The listing builds one solid part. Answer for the finished solid, in the listing's coordinates (mm). Face numbers are marked on the shaded views. A direction names the side the tool comes from. Give positions to 0.01 mm unless a question says otherwise; leave off trailing zeros. Write each loop counter-clockwise with the first axis right and the second up, starting at its lowest first coordinate (ties: lowest second). Pieces come first, ordered by that corner, then holes. Notation, with made-up numbers: (43.25, 17.25) - (91.25, 17.25) arc R26 cw to (91.25, 42.25) - close; hole circle Ø9 at (8, 49.25). An arc over 180 degrees is marked (long way). One line per question, with ' | ' between items. Start each with the question number.
1. Given P1, Ø5, axis at x = -9.5, y = -34, coming from the -Z side; P2, Ø9.5, axis at x = -35, y = -20.5, coming from the +Z side; P3, Ø2, axis at x = -29.5, z = 50.5, coming from the +Y side; P4, Ø8.5, axis at x = -37.99, y = 13.53, coming from the +Z side, each flat-ended and moving along its own axis, determine where each tip first touches the part or whether it passes through.
2. The mould has two halves that part along X. Classify the marked faces 3, 4 and 5: +X half, -X half, draft (parallel to the pull), parting line (faces both ways), or undercut.
3. A cutting plane is placed at A-A (y = 26). Determine the outline of the cut face in (x, z).
4. Find the intervals of material crossed by L1, parallel to Z at x = -31, y = -11.5; L2, parallel to Y at x = -6, z = 24; L3, parallel to X at y = -28.5, z = 17.5, in increasing order. Write a range as from..to.
5. A cutting plane is placed at D-D (x = 2). Determine the outline of the cut face in (y, z).
6. A cutting plane is placed at B-B (z = 6.5). Determine the outline of the cut face in (x, y).
7. For the marked faces 1 and 2, determine the directions among +Z, -Z, +X, -X, +Y, -Y from which every point of the face is accessible in a straight line to the end or side of a thin tool.
8. A cutting plane is placed at C-C (z = 28.5). State how many separate pieces and enclosed holes the cut face has, then the cut area to 3 significant figures.
```python
from build123d import *

# Parameters (mm, degrees)
F1_DEPTH    = 12.7
F2_R        = 9.525
F3_DEPTH    = 38.1
F4_T        = -2.54
F5_R        = 9.525
F6_DEPTH    = 63.5
F7_T        = 2.54
F7_T3_DEPTH = 12.7
F7_T5_DEPTH = 76.2
F7_T7_DEPTH = 76.2


# Not quite as in the source:
# - a shell that OpenCascade refuses in one call is made with other operations: the cavity is built on its own and cut out


with BuildPart() as f1:
    # F0 (on Top) → F1 (new body)
    with BuildSketch(Plane.XY):
        Polygon((-18.9360706136, 32.5840498031), (-57.0360706136, 32.5840498031), (-57.0360706136, -5.5159501969), (-57.0360706136, -43.6159501969), (-18.9360706136, -43.6159501969), (19.1639293864, -43.6159501969), (19.1639293864, -5.5159501969), (19.1639293864, 32.5840498031), align=None)
    extrude(amount=F1_DEPTH)

    # F2 (on face) → F3 (join)
    with BuildSketch(Plane.XY.offset(12.7)):
        with Locations((-37.9860706136, 13.5340498031)):
            Circle(F2_R)
        with Locations((0.1139293864, 13.5340498031)):
            Circle(F2_R)
        with Locations((-37.9860706136, -24.5659501969)):
            Circle(F2_R)
        with Locations((0.1139293864, -24.5659501969)):
            Circle(F2_R)
    extrude(amount=F3_DEPTH)

    # F4
    f4_openings = [f1.faces().sort_by_distance(p)[0] for p in [
        (0.113929, 13.53405, 50.8),
        (0.113929, -24.56595, 50.8),
        (-37.986071, -24.56595, 50.8),
        (-37.986071, 13.53405, 50.8),
    ]]
    offset(amount=F4_T, openings=f4_openings, kind=Kind.INTERSECTION)

    # F5 (on face) → F6 (join)
    with BuildSketch(Plane.XY.offset(12.7)):
        with Locations((-18.9360706136, -5.5159501969)):
            Circle(F5_R)
    extrude(amount=F6_DEPTH)

    # F7: shell of thickness 2.54, made by hand


with BuildPart() as f7_core1:
    # F7_t2: copy of F1
    add(f1.part)

    # the walls: a layer under each face that stays
    f7_faces = [f7_core1.faces().sort_by_distance(p)[0] for p in [
        (-18.9360706136, 30.0440498031, 6.35),
        (16.6239293864, -5.5159501969, 6.35),
        (-18.9360706136, -5.5159501969, 10.16),
        (-54.4960706136, -5.5159501969, 6.35),
        (-18.9360706136, -5.5159501969, 2.54),
        (-18.9360706136, -41.0759501969, 6.35),
        (-44.9710706136, 13.5340498031, 30.48),
        (-44.9710706136, -24.5659501969, 30.48),
        (-6.8710706136, 13.5340498031, 30.48),
        (-6.8710706136, -24.5659501969, 30.48),
        (-44.3360706136, 7.1840498031, 50.8),
        (-44.3360706136, -30.9159501969, 50.8),
        (-6.2360706136, 7.1840498031, 50.8),
        (-6.2360706136, -30.9159501969, 50.8),
        (-47.5110706136, 13.5340498031, 31.75),
        (-47.5110706136, -24.5659501969, 31.75),
        (-9.4110706136, 13.5340498031, 31.75),
        (-9.4110706136, -24.5659501969, 31.75),
        (-44.3360706136, -5.5159501969, 12.7),
        (-18.9360706136, 32.5840498031, 6.35),
        (-57.0360706136, -5.5159501969, 6.35),
        (19.1639293864, -5.5159501969, 6.35),
        (-18.9360706136, -43.6159501969, 6.35),
        (-28.4610706136, -5.5159501969, 44.45),
        (-18.9360706136, -5.5159501969, 0),
    ]]
    thicken(f7_faces, amount=-F7_T, mode=Mode.SUBTRACT)

    # F7_s4 → F7_t3 (cut)
    with BuildSketch(Plane.XY):
        Polygon((16.5985293864, 30.0186498031), (16.6239293864, 32.5840498031), (19.1639293864, 32.5840498031), (19.1639293864, 30.0440498031), align=None)
        Polygon((-54.4706706136, 30.0186498031), (-54.4960706136, 32.5840498031), (-57.0360706136, 32.5840498031), (-57.0360706136, 30.0440498031), align=None)
        Polygon((16.5985293864, -41.0505501969), (19.1639293864, -41.0759501969), (19.1639293864, -43.6159501969), (16.6239293864, -43.6159501969), align=None)
        Polygon((-54.4706706136, -41.0505501969), (-57.0360706136, -41.0759501969), (-57.0360706136, -43.6159501969), (-54.4960706136, -43.6159501969), align=None)
    extrude(amount=F7_T3_DEPTH, mode=Mode.SUBTRACT)

    # F7_s6 → F7_t5 (cut)
    with BuildSketch(Plane.YZ.offset(-57.0360706136)):
        Polygon((30.0186498031, 10.1346), (32.5840498031, 10.16), (32.5840498031, 12.7), (30.0440498031, 12.7), align=None)
        Polygon((30.0186498031, 2.5654), (32.5840498031, 2.54), (32.5840498031, 0), (30.0440498031, 0), align=None)
        Polygon((-41.0505501969, 10.1346), (-41.0759501969, 12.7), (-43.6159501969, 12.7), (-43.6159501969, 10.16), align=None)
        Polygon((-41.0505501969, 2.5654), (-41.0759501969, 0), (-43.6159501969, 0), (-43.6159501969, 2.54), align=None)
    extrude(amount=F7_T5_DEPTH, mode=Mode.SUBTRACT)

    # F7_s8 → F7_t7 (cut)
    with BuildSketch(Plane.XZ.offset(-32.5840498031)):
        Polygon((16.5985293864, 10.1346), (19.1639293864, 10.16), (19.1639293864, 12.7), (16.6239293864, 12.7), align=None)
        Polygon((16.5985293864, 2.5654), (19.1639293864, 2.54), (19.1639293864, 0), (16.6239293864, 0), align=None)
        Polygon((-54.4706706136, 10.1346), (-54.4960706136, 12.7), (-57.0360706136, 12.7), (-57.0360706136, 10.16), align=None)
        Polygon((-54.4706706136, 2.5654), (-57.0360706136, 2.54), (-57.0360706136, 0), (-54.4960706136, 0), align=None)
    extrude(amount=F7_T7_DEPTH, mode=Mode.SUBTRACT)

    # F7_s9 → F7_t10 (revolve, cut)
    with BuildSketch(Plane.XZ.offset(-13.5340498031)):
        Polygon((-28.4356706136, 12.7254), (-31.0010706136, 12.7), (-31.0010706136, 10.16), (-28.4610706136, 10.16), align=None)
    revolve(axis=Axis((-37.9860706136, 13.5340498031, 12.7), (0, 0, 1)), mode=Mode.SUBTRACT)

    # F7_s11 → F7_t12 (revolve, cut)
    with BuildSketch(Plane.XZ.offset(24.5659501969)):
        Polygon((-28.4356706136, 12.7254), (-31.0010706136, 12.7), (-31.0010706136, 10.16), (-28.4610706136, 10.16), align=None)
    revolve(axis=Axis((-37.9860706136, -24.5659501969, 12.7), (0, 0, 1)), mode=Mode.SUBTRACT)

    # F7_s13 → F7_t14 (revolve, cut)
    with BuildSketch(Plane.XZ.offset(-13.5340498031)):
        Polygon((9.6643293864, 12.7254), (7.0989293864, 12.7), (7.0989293864, 10.16), (9.6389293864, 10.16), align=None)
    revolve(axis=Axis((0.1139293864, 13.5340498031, 12.7), (0, 0, 1)), mode=Mode.SUBTRACT)

    # F7_s15 → F7_t16 (revolve, cut)
    with BuildSketch(Plane.XZ.offset(24.5659501969)):
        Polygon((9.6643293864, 12.7254), (7.0989293864, 12.7), (7.0989293864, 10.16), (9.6389293864, 10.16), align=None)
    revolve(axis=Axis((0.1139293864, -24.5659501969, 12.7), (0, 0, 1)), mode=Mode.SUBTRACT)

    # F7_s17 → F7_t18 (revolve, cut)
    with BuildSketch(Plane.XZ.offset(5.5159501969)):
        Polygon((-9.3856706136, 12.7254), (-9.4110706136, 10.16), (-11.9510706136, 10.16), (-11.9510706136, 12.7), align=None)
    revolve(axis=Axis((-18.9360706136, -5.5159501969, 12.7), (0, 0, 1)), mode=Mode.SUBTRACT)


with BuildPart() as f1_1:
    add(f1.part)

    # what is left inside the walls is the cavity
    f7_cavity = [f7_core1.part.solids().sort_by_distance(p)[0] for p in [
        (-25.895671, -5.51595, 55.033333),
    ]]
    add(f7_cavity, mode=Mode.SUBTRACT)


solid = f1_1.part
```
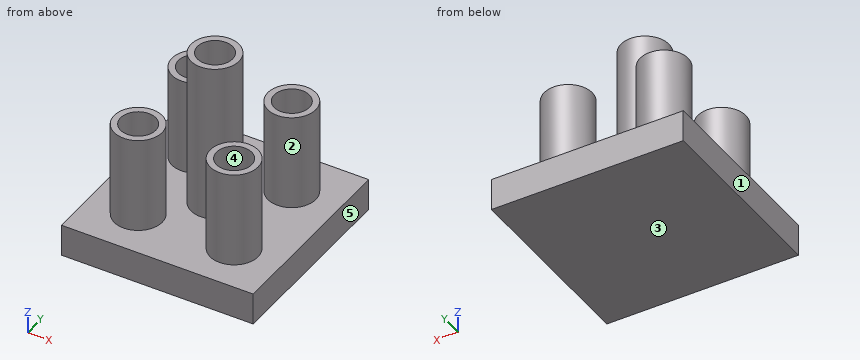
Determined:
1) P1: z = 0 | P2: z = 50.8 | P3: y = 19.42 | P4: z = 2.54
2) face 3: draft | face 4: undercut | face 5: +X half
3) outline: (-57.04, 0) - (19.16, 0) - (19.16, 12.7) - (-57.04, 12.7) - close; hole (-54.5, 2.54) - (16.62, 2.54) - (16.62, 10.16) - (-54.5, 10.16) - close
4) L1: 0..2.54, 10.16..12.7 | L2: -31.87..-27.94, -21.19..-17.26, 6.23..10.16, 16.91..20.84 | L3: -46.66..-43.76, -32.21..-29.31, -8.56..-5.66, 5.89..8.79
5) outline: (-43.62, 0) - (32.58, 0) - (32.58, 12.7) - (22.87, 12.7) - (22.87, 50.8) - (20.26, 50.8) - (20.26, 10.16) - (30.04, 10.16) - (30.04, 2.54) - (-41.08, 2.54) - (-41.08, 10.16) - (-31.29, 10.16) - (-31.29, 50.8) - (-33.9, 50.8) - (-33.9, 12.7) - (-43.62, 12.7) - close; (-17.84, 10.16) - (6.81, 10.16) - (6.81, 50.8) - (4.2, 50.8) - (4.2, 12.7) - (-15.23, 12.7) - (-15.23, 50.8) - (-17.84, 50.8) - close
6) outline: (-57.04, -43.62) - (19.16, -43.62) - (19.16, 32.58) - (-57.04, 32.58) - close; hole (-54.5, -41.08) - (16.62, -41.08) - (16.62, 30.04) - (-54.5, 30.04) - close
7) face 1: +Z, -Z, -X, +Y, -Y | face 2: +Z
8) separate pieces: 5 | enclosed holes: 5 | area: 659 mm2
